```python
from build123d import *

# Parameters (mm, degrees)
SKETCH1_R           = 3.5
SKETCH1_W           = 25.4
SKETCH1_H           = 3.175
BOSS_EXTRUDE1_DEPTH = 3.175


with BuildPart() as part:
    # Sketch1 → Boss-Extrude1 (new body)
    with BuildSketch(Plane(origin=(0, 0, 0), x_dir=(1, 0, 0), z_dir=(0, 1, 0))):
        with BuildLine():
            Line((-152.4, 19.05), (-106.95, 19.05))
            ThreePointArc((-106.95, 19.05), (-75.519103576, 6.030896424), (-62.5, -25.4))
            Line((-62.5, -25.4), (-44.642857143, -25.4))
            Line((-44.642857143, -25.4), (-26.785714286, -25.4))
            Line((-26.785714286, -25.4), (-8.928571429, -25.4))
            Line((-8.928571429, -25.4), (8.928571429, -25.4))
            Line((8.928571429, -25.4), (26.785714286, -25.4))
            Line((26.785714286, -25.4), (44.642857143, -25.4))
            Line((44.642857143, -25.4), (62.5, -25.4))
            ThreePointArc((62.5, -25.4), (75.519103576, 6.030896424), (106.95, 19.05))
            Line((106.95, 19.05), (152.4, 19.05))
            Line((152.4, 19.05), (152.4, 25.4))
            Line((152.4, 25.4), (127, 25.4))
            Line((127, 25.4), (101.6, 25.4))
            Line((101.6, 25.4), (-101.6, 25.4))
            Line((-101.6, 25.4), (-127, 25.4))
            Line((-127, 25.4), (-152.4, 25.4))
            Line((-152.4, 25.4), (-152.4, 19.05))
        make_face()
        with Locations((-44.45, -12.7)):
            Circle(SKETCH1_R, mode=Mode.SUBTRACT)
        with Locations((12.7, -12.7)):
            Circle(SKETCH1_R, mode=Mode.SUBTRACT)
        with Locations((44.45, -12.7)):
            Circle(SKETCH1_R, mode=Mode.SUBTRACT)
        with Locations((-44.45, 12.7)):
            Circle(SKETCH1_R, mode=Mode.SUBTRACT)
        with Locations((12.7, 12.7)):
            Circle(SKETCH1_R, mode=Mode.SUBTRACT)
        with Locations((44.45, 12.7)):
            Circle(SKETCH1_R, mode=Mode.SUBTRACT)
        Polygon((-44.642857143, -25.4), (-62.5, -25.4), (-62.5, -31.4), (62.5, -31.4), (62.5, -25.4), (44.642857143, -25.4), (44.642857143, -28.4), (26.785714286, -28.4), (26.785714286, -25.4), (8.928571429, -25.4), (8.928571429, -28.4), (-8.928571429, -28.4), (-8.928571429, -25.4), (-26.785714286, -25.4), (-26.785714286, -28.4), (-44.642857143, -28.4), align=None)
        with Locations((-114.3, 26.9875)):
            Rectangle(SKETCH1_W, SKETCH1_H)
        with Locations((114.3, 26.9875)):
            Rectangle(SKETCH1_W, SKETCH1_H)
    extrude(amount=BOSS_EXTRUDE1_DEPTH)


solid = part.part
```
Geometry check sheet. Reference: the model listing, model coordinates, mm. Coordinates: 2 decimals unless noted, no trailing zeros. Loops run counter-clockwise (first coordinate to the right, second up) from the corner with the lowest first, then second, coordinate; pieces in that order, holes last. Notation, with made-up numbers: (-30, 9) - (-2, 9) arc R10 cw to (-2, 22) - close; hole circle Ø3 at (-10, -4). An arc over 180 degrees is marked (long way). One line per item, written item: value. Start each with the question number.
(1) Cross-section at A-A on x = 5. Enter the section's corners in (y, z) (3 decimals), plus the area to 3 significant figures.
(2) Mould release check, pull along X, two halves, no side actions. Record for faces 1 (the cylindrical face through (75.175, 1.565, -5.683)), 2 (the cylindrical face through (-47, 1.6, -15.1)), 3 (the flat face through (-2, 0, -6)): released by +X, released by -X, zero draft, split by the parting line, or undercut.
(3) Cross-section at B-B on z = 12.7. Enter the section's corners in (x, y) (3 decimals).
(4) Cross-section at D-D on x = 114. Enter the section's corners in (y, z) (3 decimals).
(5) Material ranges on line 1 (Z direction, x = 12.7, y = 1.4); line 2 (X direction, y = 0.5, z = 26.5); line 3 (Z direction, x = -44.45, y = 0.9), recorded low to high. Write a range as [from, to].
(6) Cross-section at C-C on y = 2. Count the separate pieces of the cut face and the enclosed holes in it, plus the area to 3 significant figures.
(7) Depth check by flat-ended pin: P1, Ø0.9, axis at y = 1, z = 27, coming from the +X side; P2, Ø1, axis at x = 144.5, y = 2, coming from the -Z side; P3, Ø1.5, axis at y = 2, z = 26.5, coming from the -X side. Enter the tip coordinate at first touch or a pass-through.
Results below:
1. outline: (0, -25.4) - (3.175, -25.4) - (3.175, 25.4) - (0, 25.4) - close; (0, 28.4) - (3.175, 28.4) - (3.175, 31.4) - (0, 31.4) - close
1. area: 171 mm2
2. face 1: released by +X
2. face 2: undercut
2. face 3: zero draft
3. outline: (-64.353, 0) - (-47.95, 0) - (-47.95, 3.175) - (-64.353, 3.175) - close; (-40.95, 0) - (9.2, 0) - (9.2, 3.175) - (-40.95, 3.175) - close; (16.2, 0) - (40.95, 0) - (40.95, 3.175) - (16.2, 3.175) - close; (47.95, 0) - (64.353, 0) - (64.353, 3.175) - (47.95, 3.175) - close
4. outline: (0, -28.575) - (3.175, -28.575) - (3.175, -19.05) - (0, -19.05) - close
5. line 1: z = [-25.4, -16.2], [-9.2, 9.2], [16.2, 31.4]
5. line 2: x = [-62.5, -44.64], [-26.79, -8.93], [8.93, 26.79], [44.64, 62.5]
5. line 3: z = [-25.4, -16.2], [-9.2, 9.2], [16.2, 25.4], [28.4, 31.4]
6. separate pieces: 1
6. enclosed holes: 9
6. area: 8,860 mm2
7. P1: stops at x = 62.5
7. P2: stops at z = -25.4
7. P3: stops at x = -62.5
